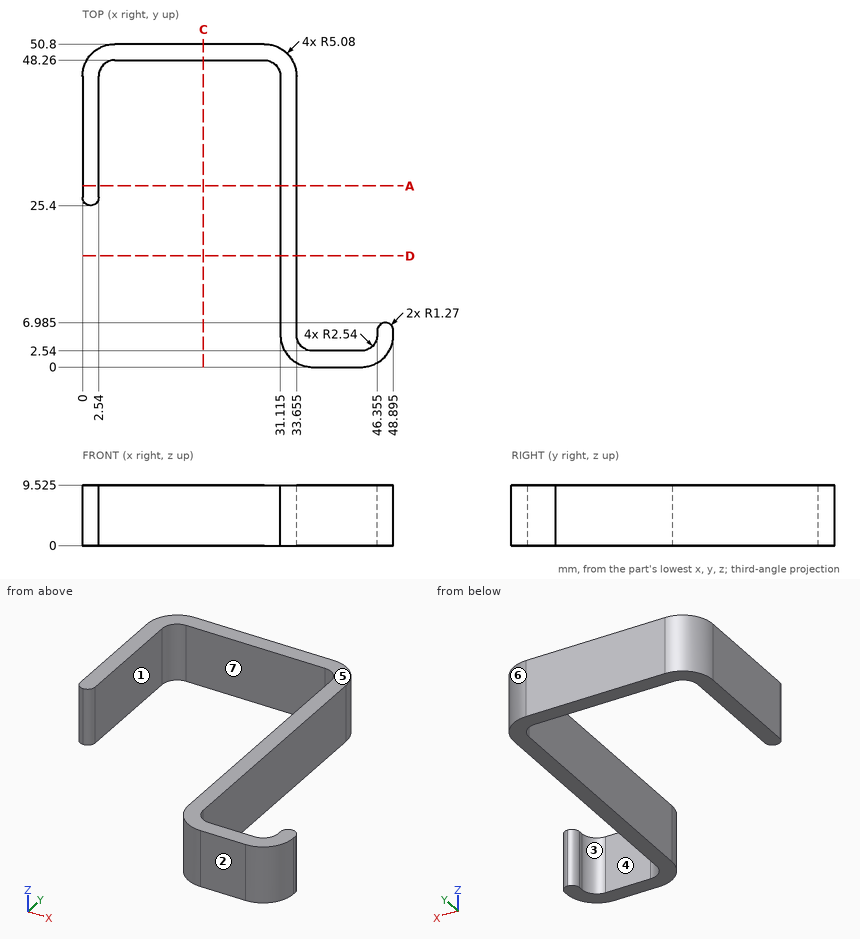
Print and shaded views of the part. All mm, measured from the part's lowest x, y and z. A direction names the side the tool comes from. Coordinates: 2 decimals unless noted, no trailing zeros. Write each loop counter-clockwise with the first axis right and the second up, starting at its lowest first coordinate (ties: lowest second). Pieces come first, ordered by that corner, then holes.
(1) 3-axis set-ups, long thin cutter, end or side, ignore diameter. For the marked faces 1, 2 and 3: which of +Z, -Z, +X, -X, +Y, -Y reach the whole face in a straight line?
(2) Cut at D-D, the plane y = 17.5. List the corners of the cut face in (x, z) (3 decimals), and give its area (3 significant figures).
(3) Cut at C-C, the plane x = 19. List the corners of the cut face in (y, z) (3 decimals), and give its area (3 significant figures).
(4) Two-plate mould, pull along X, no slides. Class the marked faces 4, 5, 6 and 7: +X half, -X half, draft (parallel to the pull), parting line (faces both ways), or undercut.
(5) Cut at A-A, the plane y = 28.5. List the corners of the cut face in (x, z) (3 decimals).
(6) Drill centre lines: probe 1 along X at (y, z) = (32, 7.25) (3 decimals); probe 2 along Y at (x, z) = (27, 5.5); probe 3 along X at (y, z) = (16, 3) (3 decimals). Where is each one in solid material? Low to high.
(7) Flat gauge pin, fed straight in: pin 1 (1 mm diameter, centred on y = 18.5, z = 6.5, fed in from +X) (3 decimals). Where does the tip first touch, or does it go through?
Geometry says:
1. face 1: +Z, -Z, -Y
1. face 2: +Z, -Z, +X, -X, -Y
1. face 3: +Z, -Z, +Y
2. outline: (31.115, 0) - (33.655, 0) - (33.655, 9.525) - (31.115, 9.525) - close
2. area: 24.2 mm2
3. outline: (48.26, 0) - (50.8, 0) - (50.8, 9.525) - (48.26, 9.525) - close
3. area: 24.2 mm2
4. face 4: undercut
4. face 5: draft
4. face 6: +X half
4. face 7: undercut
5. outline: (0, 0) - (2.54, 0) - (2.54, 9.525) - (0, 9.525) - close; (31.115, 0) - (33.655, 0) - (33.655, 9.525) - (31.115, 9.525) - close
6. probe 1: x = 0 to 2.54, 31.115 to 33.655
6. probe 2: y = 48.26 to 50.8
6. probe 3: x = 31.115 to 33.655
7. pin 1: stops at x = 33.655
